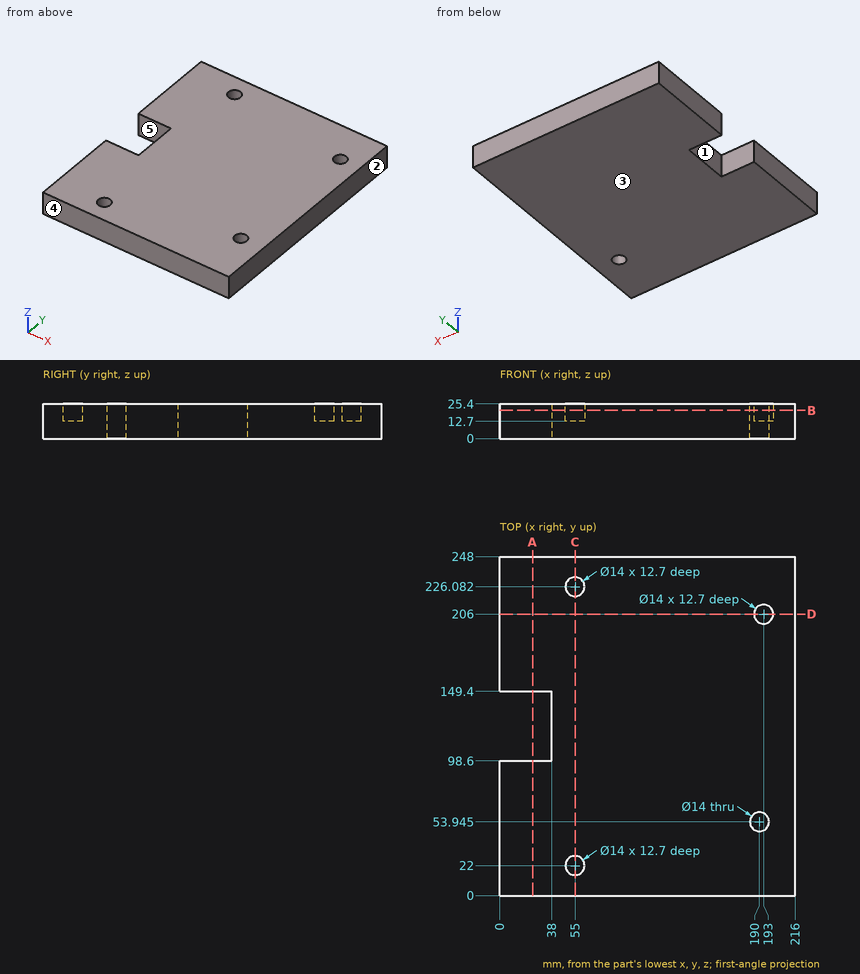
Geometry check sheet. Reference: drawing and pictorial views, mm from the part's lowest x, y, z. A direction names the side the tool comes from. Coordinates: 2 decimals unless noted, no trailing zeros. Loops run counter-clockwise (first coordinate to the right, second up) from the corner with the lowest first, then second, coordinate; pieces in that order, holes last. Notation, with made-up numbers: (6, 35.25) -> (26, 35.25) arc R12 cw to (26, 46.25) -> close; hole circle Ø8 at (60.25, 83.25). An arc over 180 degrees is marked (long way). Write item = value, one per line. Start each with the question number.
1. Section check D-D on y = 206. Record the cut outline in (x, z).
2. Section check C-C on x = 55. Record the cut outline in (y, z), then the cut area to 3 significant figures.
3. Section check B-B on z = 20.75. Record the cut outline in (x, y) (1 decimal).
4. Depth check by flat-ended pin: P1, Ø12.5, axis at x = 190, y = 53.95, coming from the -Z side; P2, Ø3, axis at y = 215, z = 16, coming from the -X side. Enter the tip coordinate at first touch or a pass-through.
5. Draft check along Y on the marked faces 3, 4 and 5. Enter one of: released by +Y, released by -Y, zero draft, split by the parting line, or undercut.
6. Tool access check on the marked faces 1 and 2. Record the directions out of +Z, -Z, +X, -X, +Y, -Y that give a thin tool (end or side, any length) a straight path to the whole face; none if there is none.
7. Section check A-A on x = 24. Record the cut outline in (y, z), then the cut area to 3 significant figures.
8. Material ranges on line 1 (Y direction, x = 55, z = 19.25); line 2 (X direction, y = 129, z = 13.5); line 3 (Y direction, x = 27.5, z = 17.5), recorded low to high.
Responses:
q1.outline = (0, 0) -> (216, 0) -> (216, 25.4) -> (200, 25.4) -> (200, 12.7) -> (186, 12.7) -> (186, 25.4) -> (0, 25.4) -> close
q2.outline = (0, 0) -> (248, 0) -> (248, 25.4) -> (233.08, 25.4) -> (233.08, 12.7) -> (219.08, 12.7) -> (219.08, 25.4) -> (29, 25.4) -> (29, 12.7) -> (15, 12.7) -> (15, 25.4) -> (0, 25.4) -> close
q2.area = 5,940 mm2
q3.outline = (0, 0) -> (216, 0) -> (216, 248) -> (0, 248) -> (0, 149.4) -> (38, 149.4) -> (38, 98.6) -> (0, 98.6) -> close; hole circle Ø14 at (55, 22); hole circle Ø14 at (55, 226.1); hole circle Ø14 at (190, 53.9); hole circle Ø14 at (193, 206)
q4.P1 = through
q4.P2 = 0
q5.face_3 = zero draft
q5.face_4 = released by -Y
q5.face_5 = undercut
q6.face_1 = +Z, -Z, -X
q6.face_2 = +Z, -Z, +X, +Y, -Y
q7.outline = (0, 0) -> (98.6, 0) -> (98.6, 25.4) -> (0, 25.4) -> close; (149.4, 0) -> (248, 0) -> (248, 25.4) -> (149.4, 25.4) -> close
q7.area = 5,010 mm2
q8.line_1 = 0 to 15, 29 to 219.08, 233.08 to 248
q8.line_2 = 38 to 216
q8.line_3 = 0 to 98.6, 149.4 to 248
